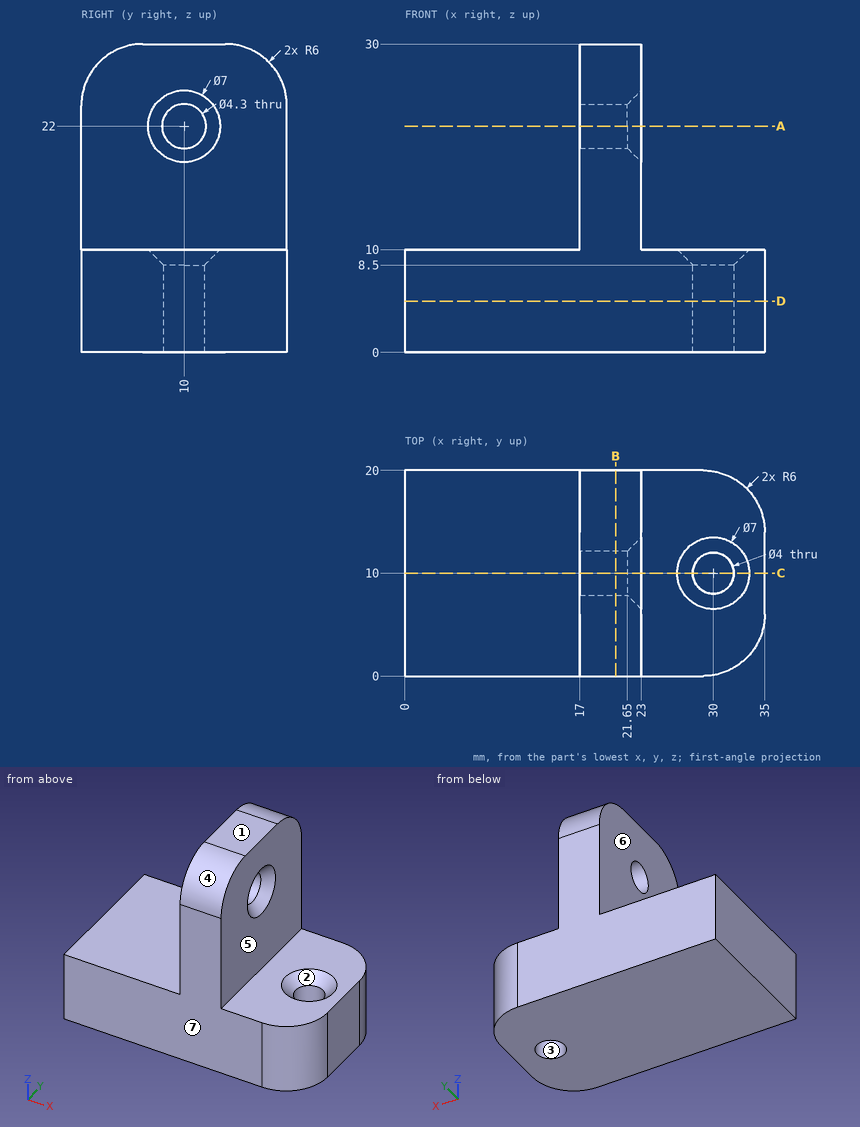
Study the drawing (mm; zero at the part's minimum x, y, z) and answer. A direction names the side the tool comes from. Give positions to 0.01 mm unless a question says otherwise; leave off trailing zeros. Loops run counter-clockwise (first coordinate to the right, second up) from the corner with the lowest first, then second, coordinate; pieces in that order, holes last. Notation, with made-up numbers: M 58.25,85 L 92.25,85 A3 cw 92.25,90 Z; hole C -29.5,53.25 d7. An arc over 180 degrees is marked long. One line per item, written item: value. Start each with the question number.
1. Each of these flat-tipped pins is pushed along its axis until it touches: P1, Ø1.5, axis at x = 17, y = 2.5, coming from the +Z side; P2, Ø12, axis at y = 2.5, z = 24.5, coming from the +X side; P3, Ø1, axis at y = 6, z = 14, coming from the -X side. Where does it stop, or does it pass through?
2. Find section B-B (x = 20.5). Give the vertices of the cut face in (y, z), and give its area (3 significant figures).
3. Find the intervals of material crossed by probe 1 along X at (y, z) = (10, 6); probe 2 along Z at (x, y) = (18.8, 10); probe 3 along X at (y, z) = (1.5, 19.5), in increasing order.
4. Determine the mould class of the marked faces 1, 2, 3 and 4 for opening direction Y: released by +Y, released by -Y, zero draft, split by the parting line, or undercut.
5. Find section C-C (y = 10). Give the vertices of the cut face in (x, z), and give its area (3 significant figures).
6. Which of the six approach directions +Z, -Z, +X, -X, +Y, -Y give full straight-line access (tool end or side, diameter ignored) to the marked faces 5, 6 and 7?
7. Find section A-A (z = 22). Give the vertices of the cut face in (x, y), and give its area (3 significant figures).
8. Find section D-D (z = 5). Give the vertices of the cut face in (x, y).
Reported:
1. P1: stops at z = 29.33
1. P2: stops at x = 23
1. P3: stops at x = 17
2. outline: M 0,0 L 20,0 L 20,24 A6 ccw 14,30 L 6,30 A6 ccw 0,24 Z; hole C 10,22 d4.3
2. area: 570 mm²
3. probe 1: x = 0 to 28, 32 to 35
3. probe 2: z = 0 to 19.85, 24.15 to 30
3. probe 3: x = 17 to 23
4. face 1: zero draft
4. face 2: undercut
4. face 3: undercut
4. face 4: released by -Y
5. outline: M 0,0 L 28,0 L 28,8.5 L 26.5,10 L 23,10 L 23,18.5 L 21.65,19.85 L 17,19.85 L 17,10 L 0,10 Z; M 17,24.15 L 21.65,24.15 L 23,25.5 L 23,30 L 17,30 Z; M 32,0 L 35,0 L 35,10 L 33.5,10 L 32,8.5 Z
5. area: 400 mm²
6. face 5: +Z, +X, +Y, -Y
6. face 6: +Z, -X, +Y, -Y
6. face 7: +Z, -Z, +X, -X, -Y
7. outline: M 17,0 L 23,0 L 23,6.5 L 21.65,7.85 L 17,7.85 Z; M 17,12.15 L 21.65,12.15 L 23,13.5 L 23,20 L 17,20 Z
7. area: 92.4 mm²
8. outline: M 0,0 L 29,0 A6 ccw 35,6 L 35,14 A6 ccw 29,20 L 0,20 Z; hole C 30,10 d4
